Part model, mm, in its own coordinate system. A direction names the side the tool comes from. Coordinates: 2 decimals unless noted, no trailing zeros. Order: outer loops, then holes, each group sorted by start corner. A loop starts at its lowest first (then second) coordinate and runs counter-clockwise, first axis right, second up.
```python
from build123d import *

# Parameters (mm, degrees)
F1_DEPTH = 101.6
F2_R     = 1.8288
F3_DEPTH = 3.175


with BuildPart() as f1:
    # F0 (on Top) → F1 (new body)
    with BuildSketch(Plane.XY):
        with BuildLine():
            Line((29.136266, -4.530016), (29.136266, 24.044984))
            ThreePointArc((29.136266, 24.044984), (26.686291, 27.711631), (22.361186, 26.851314))
            Line((22.361186, 26.851314), (-2.245064, 2.245064))
            ThreePointArc((-2.245064, 2.245064), (-3.105381, -2.080041), (0.561266, -4.530016))
            Line((0.561266, -4.530016), (29.136266, -4.530016))
        make_face()
        with BuildLine():
            Line((25.961266, -1.355016), (0.561266, -1.355016))
            ThreePointArc((0.561266, -1.355016), (-0.172063, -0.865021), (0, 0))
            Line((0, 0), (24.60625, 24.60625))
            ThreePointArc((24.60625, 24.60625), (25.471271, 24.778313), (25.961266, 24.044984))
            Line((25.961266, 24.044984), (25.961266, -1.355016))
        make_face(mode=Mode.SUBTRACT)
    extrude(amount=F1_DEPTH)

    # F2 (on face) → F3 (cut, through all)
    with BuildSketch(Plane(origin=(25.961266, 0, 0), x_dir=(0, -1, 0), z_dir=(-1, 0, 0))):
        with Locations((-20.076234, 5.55625)):
            Circle(F2_R)
        with Locations((-2.613734, 5.55625)):
            Circle(F2_R)
        with Locations((-2.613734, 96.04375)):
            Circle(F2_R)
        with Locations((-20.076234, 96.04375)):
            Circle(F2_R)
    extrude(amount=-F3_DEPTH, mode=Mode.SUBTRACT)


solid = f1.part
```
(1) Drop flat-ended pins along their axis: pin 1 (3 mm diameter, centred on y = 20.08, z = 5.56, fed in from -X); pin 2 (3 mm diameter, centred on y = 2.61, z = 5.56, fed in from -X); pin 3 (7.5 mm diameter, centred on y = 6.5, z = 33.5, fed in from -X). Give the stop position or say it passes through.
(2) Slice it at C-C, the plane x = 3. Give the cut face in (y, z), then the cut area to 3 significant figures.
(3) Probe line 1 (X direction, y = 18, z = 76.5); line 2 (X direction, y = 5.5, z = 52); line 3 (Y direction, x = 18, z = 35). List the from-to ranges inside material, lowest first.
(4) Slice it at A-A, the plane z = 87. Give the cut face in (x, y).
(5) Slice it at B-B, the plane y = 6.5. Give the cut face in (x, z), then the cut area to 3 significant figures.
(6) Tool access for faces 4 (the face through (12, 12, 50)), 5 (the face through (12.79, 13.02, 101.6)), 6 (the face through (27.527, 19.093, 97.586)): list every direction of +Z, -Z, +X, -X, +Y, -Y with a clear straight run to the whole face (end or side of a thin tool).
(7) Slice it at D-D, the plane x = 27.5. Give the cut face in (y, z).
(8) Pull direction Y, two halves, no side cores. Call faces 1 (the face through (27.527, 18.387, 4.856)), 2 (the face through (29.136, 10, 50)), 3 (the face through (-3.13, -2.02, 50.09)): +Y half, -Y half, draft (parallel to the pull), parting line (faces both ways), or undercut.
Here are the results:
1. pin 1: stops at x = 14.09
1. pin 2: stops at x = -3.04
1. pin 3: stops at x = -1.74
2. outline: (-4.53, 0) - (-1.36, 0) - (-1.36, 101.6) - (-4.53, 101.6) - close; (3, 0) - (7.49, 0) - (7.49, 101.6) - (3, 101.6) - close
2. area: 779 mm2
3. line 1: x = 13.51 to 18, 25.96 to 29.14
3. line 2: x = 1.01 to 5.5, 25.96 to 29.14
3. line 3: y = -4.53 to -1.36, 18 to 22.49
4. outline: (-2.25, 2.25) arc R3.97 ccw to (0.56, -4.53) - (29.14, -4.53) - (29.14, 24.04) arc R3.97 ccw to (22.36, 26.85) - close; hole (0, 0) arc R0.79 ccw to (0.56, -1.36) - (25.96, -1.36) - (25.96, 24.04) arc R0.79 ccw to (24.61, 24.61) - close
5. outline: (2.01, 0) - (6.5, 0) - (6.5, 101.6) - (2.01, 101.6) - close; (25.96, 0) - (29.14, 0) - (29.14, 101.6) - (25.96, 101.6) - close
5. area: 779 mm2
6. face 4: +Z, -Z
6. face 5: +Z, +X, -X, +Y, -Y
6. face 6: +X
7. outline: (-4.53, 0) - (27.26, 0) - (27.26, 101.6) - (-4.53, 101.6) - close; hole circle Ø3.66 at (2.61, 5.56); hole circle Ø3.66 at (2.61, 96.04); hole circle Ø3.66 at (20.08, 5.56); hole circle Ø3.66 at (20.08, 96.04)
8. face 1: undercut
8. face 2: draft
8. face 3: parting line
